Source: CAD feature listing. Evaluate the final solid. Frame: model axes, mm. A direction names the side the tool comes from. Give positions to 0.01 mm unless a question says otherwise; leave off trailing zeros. Order: outer loops, then holes, each group sorted by start corner. A loop starts at its lowest first (then second) coordinate and runs counter-clockwise, first axis right, second up. Notation, with made-up numbers: M -35.75,-36.5 L -16.75,-36.5 A9 ccw -16.75,-29.5 Z; hole C -30,82 d2. An arc over 180 degrees is marked long. Return JSON: item names as keys, results as strings.
from build123d import *

# Parameters (mm, degrees)
F1_DEPTH = 101.6
F2_R     = 2.75
F3_DEPTH = 25
F4_R     = 3
F5_DEPTH = 30


with BuildPart() as f1:
    # F0 (on Right) → F1 (new body)
    with BuildSketch(Plane.YZ):
        Polygon((-134.565088, 133.698854), (-134.565088, 118.698854), (-34.565088, 118.698854), (-34.565088, 13.698854), (-19.565088, 13.698854), (-19.565088, 133.698854), align=None)
    extrude(amount=F1_DEPTH)

    # F2 (on face) → F3 (join)
    with BuildSketch(Plane.XZ.offset(34.565088)):
        with Locations((9.499623, 23.894975)):
            Circle(F2_R)
        with Locations((21.199623, 23.894975)):
            Circle(F2_R)
        with Locations((32.899623, 23.894975)):
            Circle(F2_R)
        with Locations((44.599623, 23.894975)):
            Circle(F2_R)
        with Locations((56.299623, 23.894975)):
            Circle(F2_R)
        with Locations((67.999623, 23.894975)):
            Circle(F2_R)
        with Locations((79.699623, 23.894975)):
            Circle(F2_R)
        with Locations((91.399623, 23.894975)):
            Circle(F2_R)
        with Locations((9.499623, 76.211095)):
            Circle(F2_R)
        with Locations((21.199617, 76.199905)):
            Circle(F2_R)
        with Locations((32.899612, 76.188715)):
            Circle(F2_R)
        with Locations((44.599606, 76.177524)):
            Circle(F2_R)
        with Locations((56.299601, 76.166334)):
            Circle(F2_R)
        with Locations((67.999596, 76.155144)):
            Circle(F2_R)
        with Locations((79.69959, 76.143954)):
            Circle(F2_R)
        with Locations((91.399585, 76.132764)):
            Circle(F2_R)
    extrude(amount=F3_DEPTH)

    # F4 (on face) → F5 (cut)
    with BuildSketch(Plane(origin=(0, 0, 118.698854), x_dir=(1, 0, 0), z_dir=(0, 0, -1))):
        with Locations((9.251543, 68.155386)):
            Circle(F4_R)
        with Locations((20.951543, 68.155386)):
            Circle(F4_R)
        with Locations((32.651543, 68.155386)):
            Circle(F4_R)
        with Locations((44.351543, 68.155386)):
            Circle(F4_R)
        with Locations((56.051543, 68.155386)):
            Circle(F4_R)
        with Locations((67.751543, 68.155386)):
            Circle(F4_R)
        with Locations((79.451543, 68.155386)):
            Circle(F4_R)
        with Locations((91.151543, 68.155386)):
            Circle(F4_R)
        with Locations((9.251543, 84.600329)):
            Circle(F4_R)
        with Locations((20.951543, 84.600329)):
            Circle(F4_R)
        with Locations((32.651543, 84.600329)):
            Circle(F4_R)
        with Locations((44.351543, 84.600329)):
            Circle(F4_R)
        with Locations((56.051543, 84.600329)):
            Circle(F4_R)
        with Locations((67.751543, 84.600329)):
            Circle(F4_R)
        with Locations((79.451543, 84.600329)):
            Circle(F4_R)
        with Locations((91.151543, 84.600329)):
            Circle(F4_R)
        with Locations((9.251543, 98.667689)):
            Circle(F4_R)
        with Locations((20.951543, 98.667689)):
            Circle(F4_R)
        with Locations((32.651543, 98.667689)):
            Circle(F4_R)
        with Locations((44.351543, 98.667689)):
            Circle(F4_R)
        with Locations((56.051543, 98.667689)):
            Circle(F4_R)
        with Locations((67.751543, 98.667689)):
            Circle(F4_R)
        with Locations((79.451543, 98.667689)):
            Circle(F4_R)
        with Locations((91.151543, 98.667689)):
            Circle(F4_R)
    extrude(amount=-F5_DEPTH, mode=Mode.SUBTRACT)


solid = f1.part
1. Draft query along Y for faces 1 (the face through (56, -59.565, 76)), 2 (the face through (69.36, -101.2, 126.09)), 3 (the face through (50, -27, 13.699)). Return one class per face: pulls with the +Y half, pulls with the -Y half, needs draft (parallel to the pull), parting line crosses it, or undercut.
Evaluation:
{"face 1": "pulls with the -Y half", "face 2": "undercut", "face 3": "needs draft"}
2. Section query A-A (x = 21). Return loops of the section in (y, z) (3 decimals), then the cut area to 3 significant figures.
Evaluation:
{"outline": "M -134.565,118.699 L -101.667,118.699 L -101.667,133.699 L -134.565,133.699 Z; M -95.668,118.699 L -87.6,118.699 L -87.6,133.699 L -95.668,133.699 Z; M -81.601,118.699 L -71.155,118.699 L -71.155,133.699 L -81.601,133.699 Z; M -65.156,118.699 L -34.565,118.699 L -34.565,78.943 L -59.565,78.943 L -59.565,73.457 L -34.565,73.457 L -34.565,26.638 L -59.565,26.638 L -59.565,21.152 L -34.565,21.152 L -34.565,13.699 L -19.565,13.699 L -19.565,133.699 L -65.156,133.699 Z", "area": "3,300 mm^2"}
3. Set-up query: faces 4 (the face through (57.664, -87.13, 126.094)), 5 (the face through (91, -59.565, 24)), 6 (the face through (94, -47, 23)). Return all of +Z, -Z, +X, -X, +Y, -Y with unobstructed straight access to the full face (end or side cutting, diameter ignored); none if empty.
Evaluation:
{"face 4": "+Z, -Z", "face 5": "-Z, +X, -X, -Y", "face 6": "-Y"}
4. Section query C-C (y = -93.5). Return loops of the section in (x, z), then the cut area to 3 significant figures.
Evaluation:
{"outline": "M 0,118.7 L 101.6,118.7 L 101.6,133.7 L 0,133.7 Z", "area": "1,520 mm^2"}
5. Section query D-D (x = 68.5). Return loops of the section in (y, z), then the cut area to 3 significant figures.
Evaluation:
{"outline": "M -134.57,118.7 L -101.57,118.7 L -101.57,133.7 L -134.57,133.7 Z; M -95.76,118.7 L -87.51,118.7 L -87.51,133.7 L -95.76,133.7 Z; M -81.7,118.7 L -71.06,118.7 L -71.06,133.7 L -81.7,133.7 Z; M -65.25,118.7 L -34.57,118.7 L -34.57,78.86 L -59.57,78.86 L -59.57,73.45 L -34.57,73.45 L -34.57,26.6 L -59.57,26.6 L -59.57,21.19 L -34.57,21.19 L -34.57,13.7 L -19.57,13.7 L -19.57,133.7 L -65.25,133.7 Z", "area": "3,310 mm^2"}
6. Section query B-B (z = 45.5). Return loops of the section in (x, y), then the cut area to 3 significant figures.
Evaluation:
{"outline": "M 0,-34.57 L 101.6,-34.57 L 101.6,-19.57 L 0,-19.57 Z", "area": "1,520 mm^2"}
7. Ray query, probe 1 along Y at (x, z) = (30.5, 123); probe 2 along Z at (x, y) = (57, -47); probe 3 along Z at (x, y) = (37.5, -43.5). Return the intervals inside material, ascending.
Evaluation:
{"probe 1": "y = -134.57 to -100.76, -96.58 to -86.69, -82.51 to -70.25, -66.06 to -19.57", "probe 2": "z = 21.24 to 26.55, 73.51 to 78.83, 118.7 to 133.7", "probe 3": "z = 118.7 to 133.7"}
8. First-contact query: pin 1 (3 mm diameter, centred on x = 91, z = 25, fed in from -Y); pin 2 (8 mm diameter, centred on x = 58, z = 61, fed in from -Y); pin 3 (9.5 mm diameter, centred on x = 9.25, y = -68.16, fed in from -Z). Flat tips, straight axial feed; report the tip coordinate or a pass-through.
Evaluation:
{"pin 1": "stops at y = -59.57", "pin 2": "stops at y = -34.57", "pin 3": "stops at z = 118.7"}
